from build123d import *

# Parameters (mm, degrees)
CHAMFER1_SIZE = 0.254
CHAMFER2_SIZE = 0.508
CHAMFER3_SIZE = 0.508


with BuildPart() as part:
    # Sketch1 → Revolve1 (revolve)
    with BuildSketch(Plane(origin=(0, 0, 0), x_dir=(1, 0, 0), z_dir=(0, 1, 0)), mode=Mode.PRIVATE) as revolve1_sk:
        Polygon((-54.186066728, 7.169875811), (-57.996066728, 7.169875811), (-57.996066728, 6.534875811), (-42.756066728, 6.534875811), (-42.756066728, 12.884875811), (-43.518066728, 12.884875811), (-43.518066728, 8.916125811), (-54.186066728, 8.916125811), align=None)
    revolve(revolve1_sk.sketch.rotate(Axis((-57.996066728, 0, -3.359875811), (1, 0, 0)), 180), axis=Axis((-57.996066728, 0, -3.359875811), (1, 0, 0)))

    # Chamfer1
    chamfer1_edges = [part.edges().sort_by_distance(p)[0] for p in [
        (-57.996066728, 0, -7.169875811),
        (-57.996066728, 0, -6.534875811),
    ]]
    chamfer(chamfer1_edges, length=CHAMFER1_SIZE)

    # Chamfer2
    chamfer2_edges = [part.edges().sort_by_distance(p)[0] for p in [
        (-42.756066728, 0, -6.534875811),
    ]]
    chamfer(chamfer2_edges, length=CHAMFER2_SIZE)

    # Chamfer3
    chamfer3_edges = [part.edges().sort_by_distance(p)[0] for p in [
        (-42.756066728, 0, -12.884875811),
    ]]
    chamfer(chamfer3_edges, length=CHAMFER3_SIZE)


solid = part.part
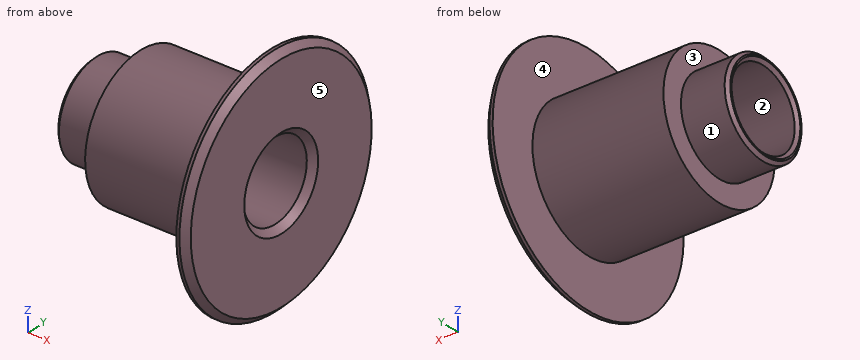
CAD build for the part. Positions are in the model's coordinates, mm. Face numbers are marked on the shaded views. A direction names the side the tool comes from. Round coordinates to 2 decimals unless told otherwise and drop trailing zeros. Loops run counter-clockwise (first coordinate to the right, second up) from the corner with the lowest first, then second, coordinate; pieces in that order, holes last.
(1) Which spindle directions (+Z, -Z, +X, -X, +Y, -Y) get a long thin tool onto all of the face, cutting with end or side? Do the marked faces 4 and 5. Say none if no direction does.
(2) Wall check: line 1 along X through (y, z) = (-3, -8.5); line 2 along Z through (x, y) = (-46, -2.5); line 3 along X through (y, z) = (-4.75, -3). Give the ranges that are in metal, low to high.
(3) Two-plate mould, pull along Z, no slides. Class the marked faces 1, 2 and 3: +Z half, -Z half, draft (parallel to the pull), parting line (faces both ways), or undercut.
(4) Cut at A-A (y = 0). Give the cut face in (x, z), plus the area to 3 significant figures.
(5) Cut at B-B (x = -55.25). Give the cut face in (y, z) (3 decimals), plus the area to 3 significant figures.
(6) Drop flat-ended pins along their axis: pin 1 (5 mm diameter, centred on x = -55, y = -3, fed in from -Z); pin 2 (4 mm diameter, centred on x = -54, y = 6, fed in from +Z); pin 3 (1.5 mm diameter, centred on x = -55.5, z = -10.5, fed in from -Y); pin 4 (2 mm diameter, centred on y = -2.5, z = -5.5, fed in from +X). Give the stop position or say it passes through.
Findings below:
1. face 4: -X
1. face 5: +Z, -Z, +X, +Y, -Y
2. line 1: x = -43.52 to -42.76
2. line 2: z = -8.32 to -5.32, -1.4 to 1.6
2. line 3: x = -54.19 to -42.76
3. face 1: parting line
3. face 2: undercut
3. face 3: draft
4. outline: (-58, -6.92) - (-57.74, -7.17) - (-54.19, -7.17) - (-54.19, -8.92) - (-43.52, -8.92) - (-43.52, -12.88) - (-43.26, -12.88) - (-42.76, -12.38) - (-42.76, -7.04) - (-43.26, -6.53) - (-57.74, -6.53) - (-58, -6.79) - close; (-58, 0.07) - (-57.74, -0.18) - (-43.26, -0.18) - (-42.76, 0.32) - (-42.76, 5.66) - (-43.26, 6.17) - (-43.52, 6.17) - (-43.52, 2.2) - (-54.19, 2.2) - (-54.19, 0.45) - (-57.74, 0.45) - (-58, 0.2) - close
4. area: 64.7 mm2
5. outline: circle Ø7.62 at (0, -3.36); hole circle Ø6.35 at (0, -3.36)
5. area: 13.9 mm2
6. pin 1: stops at z = -8.88
6. pin 2: stops at z = 0.5
6. pin 3: passes through
6. pin 4: stops at x = -42.76
